from build123d import *

# Parameters (mm, degrees)
EXTRUDE_2_DEPTH     = 140
SKETCH_4_W          = 6
SKETCH_4_H          = 19
CUT_EXTRUDE_1_DEPTH = 1
SKETCH_3_R          = 3
EXTRUDE_4_DEPTH     = 5
CHAMFER_2_SIZE      = 1
FILLET_2_R          = 2
SKETCH_6_W          = 102
SKETCH_6_H          = 1
EXTRUDE_5_DEPTH     = 30
FILLET_3_R          = 10
SKETCH_7_W          = 2
SKETCH_7_H          = 102
EXTRUDE_6_DEPTH     = 5


with BuildPart() as part:
    # 草图2 → 凸台-拉伸2 (new body)
    with BuildSketch(Plane.XY):
        with BuildLine():
            Line((-3, 0), (3, 0))
            Line((3, 0), (3, 1))
            ThreePointArc((3, 1), (0, 4), (-3, 1))
            Line((-3, 1), (-3, 0))
        make_face()
    extrude(amount=EXTRUDE_2_DEPTH)

    # 草图4 → 切除-拉伸1 (cut)
    with BuildSketch(Plane.XZ):
        with Locations((0, 130.5)):
            Rectangle(SKETCH_4_W, SKETCH_4_H)
        with Locations((0, 9.5)):
            Rectangle(SKETCH_4_W, SKETCH_4_H)
    extrude(amount=-CUT_EXTRUDE_1_DEPTH, mode=Mode.SUBTRACT)

    # 草图3 → 凸台-拉伸4 (add)
    with BuildSketch(Plane.XZ.offset(-1)):
        with Locations(Location((0, 131, 0), (0, 0, 180))):
            Circle(SKETCH_3_R)
        with Locations(Location((0, 9, 0), (0, 0, 180))):
            Circle(SKETCH_3_R)
    extrude(amount=EXTRUDE_4_DEPTH)

    # 倒角2
    chamfer_2_edges = [part.edges().sort_by_distance(p)[0] for p in [
        (3, -4, 131),
        (3, -4, 9),
    ]]
    chamfer(chamfer_2_edges, length=CHAMFER_2_SIZE)

    # 圆角2
    fillet_2_edges = [part.edges().sort_by_distance(p)[0] for p in [
        (0, 4, 140),
        (0, 4, 0),
    ]]
    fillet(fillet_2_edges, radius=FILLET_2_R)

    # 草图6 → 凸台-拉伸5 (add)
    with BuildSketch(Plane(origin=(3, 0, 0), x_dir=(0, 0, -1), z_dir=(1, 0, 0))):
        with Locations((-70, 0.5)):
            Rectangle(SKETCH_6_W, SKETCH_6_H)
    extrude(amount=EXTRUDE_5_DEPTH)

    # 圆角3
    fillet_3_edges = [part.edges().sort_by_distance(p)[0] for p in [
        (33, 0.5, 121),
        (33, 0.5, 19),
    ]]
    fillet(fillet_3_edges, radius=FILLET_3_R)

    # 草图7 → 凸台-拉伸6 (add)
    with BuildSketch(Plane.XZ):
        with Locations((-2, 70)):
            Rectangle(SKETCH_7_W, SKETCH_7_H)
    extrude(amount=EXTRUDE_6_DEPTH)


solid = part.part
Part model, mm, in its own coordinate system. A direction names the side the tool comes from. Give positions to 0.01 mm unless a question says otherwise; leave off trailing zeros. Order: outer loops, then holes, each group sorted by start corner. A loop starts at its lowest first (then second) coordinate and runs counter-clockwise, first axis right, second up. Notation, with made-up numbers: (81.25, -4) - (112.25, -4) arc R32 ccw to (112.25, 26) - close; hole circle Ø2 at (-1.75, 55.25). An arc over 180 degrees is marked (long way). Use a Markdown table: item, result.
1) Probe L1, parallel to Y at x = 19, z = 64; L2, parallel to Y at x = 0, z = 51; L3, parallel to X at y = -1.5, z = 41. List the from-to ranges inside material, lowest first. Write a range as from..to.
Checked values:
| item | result |
|---|---|
| L1 | 0..1 |
| L2 | 0..4 |
| L3 | -3..-1 |
2) Saw through at A-A on z = 32. List the corners of the cut face in (x, y).
Checked values:
| item | result |
|---|---|
| outline | (-3, -5) - (-1, -5) - (-1, 0) - (33, 0) - (33, 1) - (3, 1) arc R3 ccw to (-3, 1) - close |
3) Saw through at C-C on x = 27. List the corners of the cut face in (y, z), plus the area to 3 significant figures.
Checked values:
| item | result |
|---|---|
| outline | (0, 19.83) - (1, 19.83) - (1, 120.17) - (0, 120.17) - close |
| area | 100 mm² |
4) Flat gauge pins, fed straight in: P1, Ø5, axis at x = 0, z = 124.5, coming from the -Y side; P2, Ø6.5, axis at x = 0, z = 12.5, coming from the -Y side; P3, Ø4, axis at x = 22, z = 43, coming from the -Y side. Where does each tip first touch, or does it go through?
Checked values:
| item | result |
|---|---|
| P1 | y = 1 |
| P2 | y = -4 |
| P3 | y = 0 |
5) Saw through at B-B on x = 14. List the corners of the cut face in (y, z), plus the area to 3 significant figures.
Checked values:
| item | result |
|---|---|
| outline | (0, 19) - (1, 19) - (1, 121) - (0, 121) - close |
| area | 102 mm² |
6) 3-axis set-ups, long thin cutter, end or side, ignore diameter. For faces 1 (the cylindrical face through (0, 4, 69)), 2 (the cylindrical face through (-1.61, -0.97, 128.47)), 3 (the flat face through (7.1, 0.5, 19)), 4 (the flat face through (0, -4, 9)), 5 (the flat face through (-3, -2, 69)): which of +Z, -Z, +X, -X, +Y, -Y reach the whole face in a straight line?
Checked values:
| item | result |
|---|---|
| face 1 | +Z, -Z, +Y |
| face 2 | -Y |
| face 3 | +X, -X, -Y |
| face 4 | -Z, +X, -X, -Y |
| face 5 | +Z, -Z, -X, +Y, -Y |
7) Two-plate mould, pull along Z, no slides. Class faces 6 (the flat face through (-1, -2, 69)), 7 (the cylindrical face through (29.99, 0.51, 21.85)), 8 (the cylindrical face through (29.99, 0.51, 118.15)), 9 (the flat face through (0, -4, 131)): +Z half, -Z half, draft (parallel to the pull), parting line (faces both ways), or undercut.
Checked values:
| item | result |
|---|---|
| face 6 | undercut |
| face 7 | -Z half |
| face 8 | +Z half |
| face 9 | draft |
